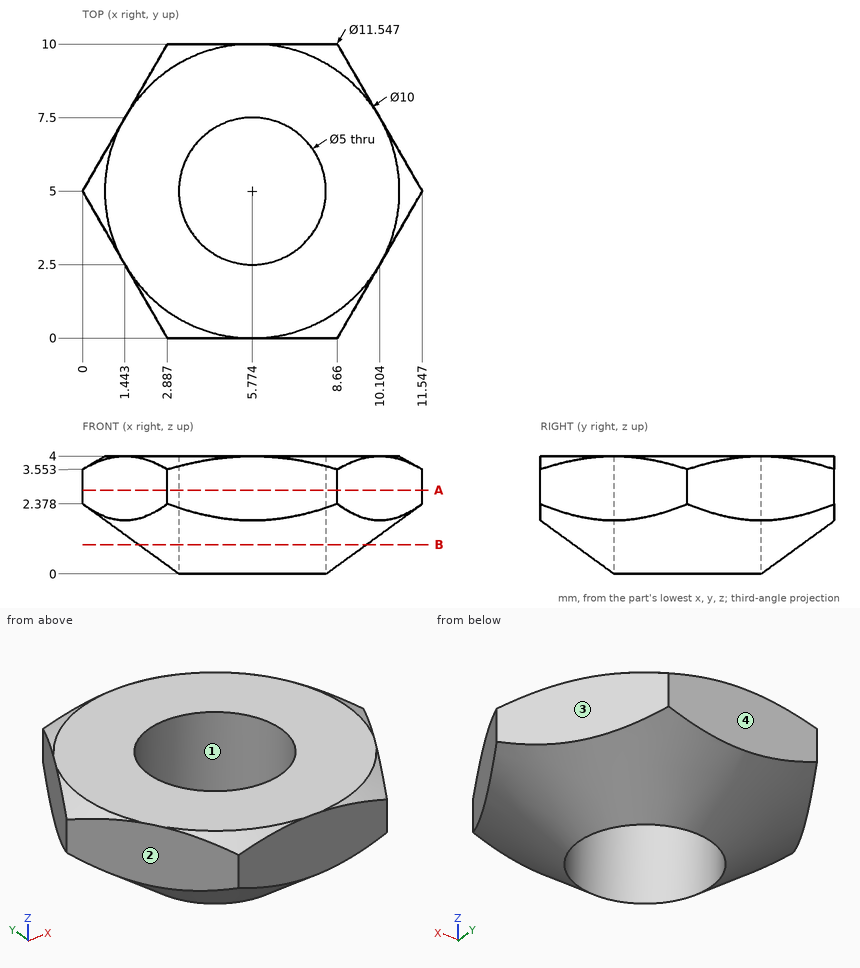
Input: dimensioned drawing with shaded views. Units: mm. Origin: part minimum x, y, z. Coordinates: 2 decimals unless noted, no trailing zeros. Write each loop counter-clockwise with the first axis right and the second up, starting at its lowest first coordinate (ties: lowest second). Pieces come first, ordered by that corner, then holes. Notation, with made-up numbers: M -12,-40 L 16,-40 A17 cw 16,-20 Z; hole C 20,20 d11. An arc over 180 degrees is marked long. Use a Markdown table: item, result.
1) Section B-B, the plane z = 1. Output: boundary loops of the cut face in (x, y).
Conclusion:
| item | result |
|---|---|
| outline | C 5.77,5 d7.75; hole C 5.77,5 d5 |
2) First-contact query: pin 1 Ø1.5 at (x, z) = (8, 1.5) entering from -Y. Flat tip, straight axial feed; report the tip coordinate or a pass-through.
Conclusion:
| item | result |
|---|---|
| pin 1 | stops at y = 0 |
3) Ray query, L1, parallel to Y at x = 7.75, z = 1.35 (1 decimal); L2, parallel to X at y = 5, z = 1.35 (1 decimal); L3, parallel to Y at x = 6, z = 1.55 (1 decimal). Return the intervals inside material, ascending.
Conclusion:
| item | result |
|---|---|
| L1 | y = 1.1 to 3.5, 6.5 to 8.9 |
| L2 | x = 1.4 to 3.3, 8.3 to 10.1 |
| L3 | y = 0.4 to 2.5, 7.5 to 9.6 |
4) Mould query, pull axis X, two halves, no side actions, for the marked faces 1, 2, 3 and 4. Classes: pulls with the +X half, pulls with the -X half, needs draft (parallel to the pull), parting line crosses it, or undercut.
Conclusion:
| item | result |
|---|---|
| face 1 | undercut |
| face 2 | pulls with the -X half |
| face 3 | pulls with the +X half |
| face 4 | needs draft |
5) Section A-A, the plane z = 2.85. Output: boundary loops of the cut face in (x, y).
Conclusion:
| item | result |
|---|---|
| outline | M 0,5 L 2.89,0 L 8.66,0 L 11.55,5 L 8.66,10 L 2.89,10 Z; hole C 5.77,5 d5 |
